Could you check a few things on this drawing? It's one solid part, dimensions in mm from its lowest x, y, z. A direction names the side the tool comes from. Give positions to 0.01 mm unless a question says otherwise; leave off trailing zeros. Order: outer loops, then holes, each group sorted by start corner. A loop starts at its lowest first (then second) coordinate and runs counter-clockwise, first axis right, second up. Notation, with made-up numbers: M 72,-28.75 L 113,-28.75 A23 ccw 113,-12.75 Z; hole C -7.75,55.5 d1. An arc over 180 degrees is marked long. Use one line per item in the form item = value. Start each with the question number.
1. I want a section at C-C, the plane z = 3.5. Count the separate pieces of the cut face and the enclosed holes in it, and give its area (3 significant figures).
2. I want a section at B-B, the plane y = 8. List the corners of the cut face in (x, z) for me.
3. Will these pins go through, and if not, where does the flat tip stop? P1, Ø3, axis at x = 10, z = 3, coming from the +Y side; P2, Ø1.7, axis at x = 2, z = 3.5, coming from the +Y side; P3, Ø1.7, axis at x = 6, z = 3.5, coming from the -Y side.
4. We'd pull the mould along Z, two halves only. Please class the marked faces 4, 5 and 6: +Z half, -Z half, draft (parallel to the pull), parting line (faces both ways), or undercut.
5. I need wall thicknesses on L1, parallel to Z at x = 4, y = 5.1; L2, parallel to Y at x = 2, z = 5.75; L3, parallel to Y at x = 13, z = 1.25. Which ranges of each line are inside material? Lowest first, please.
6. I want a section at A-A, the plane x = 4. List the corners of the cut face in (y, z) for me.
7. I want a section at D-D, the plane x = 9. List the corners of the cut face in (y, z) for me.
8. For the marked faces 1, 2 and 3, which set-ups out of +Z, -Z, +X, -X, +Y, -Y let a thin tool reach every point of the face, with its end or its side?
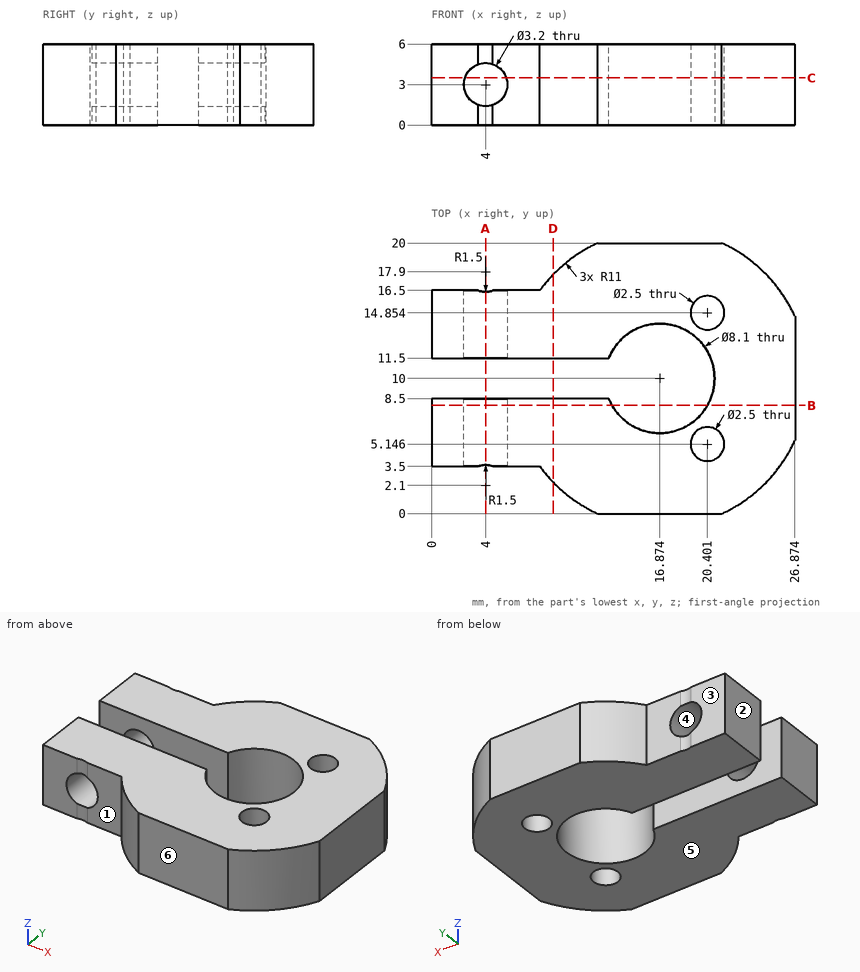
Check result:
q1.separate_pieces = 3
q1.enclosed_holes = 2
q1.area = 316 mm2
q2.outline = M 0,0 L 13.35,0 L 13.35,6 L 0,6 Z; M 20.4,0 L 26.87,0 L 26.87,6 L 20.4,6 Z; hole C 4,3 d3.2
q3.P1 = 19.6
q3.P2 = 16.5
q3.P3 = 3.5
q4.face_4 = undercut
q4.face_5 = -Z half
q4.face_6 = draft
q5.L1 = 0 to 1.4, 4.6 to 6
q5.L2 = 3.5 to 8.5, 11.5 to 16.5
q5.L3 = 0 to 8.5, 11.5 to 20
q6.outline = M 3.6,0 L 8.5,0 L 8.5,1.4 L 3.6,1.4 Z; M 3.6,4.6 L 8.5,4.6 L 8.5,6 L 3.6,6 Z; M 11.5,0 L 16.4,0 L 16.4,1.4 L 11.5,1.4 Z; M 11.5,4.6 L 16.4,4.6 L 16.4,6 L 11.5,6 Z
q7.outline = M 2.32,0 L 8.5,0 L 8.5,6 L 2.32,6 Z; M 11.5,0 L 17.68,0 L 17.68,6 L 11.5,6 Z
q8.face_1 = +Z, -Z, -X, -Y
q8.face_2 = +Z, -Z, -X, +Y, -Y
q8.face_3 = +Z, -Z, -X, +Y
